```python
from build123d import *

# Parameters (mm, degrees)
SM_BASE_FLANGE_1_DEPTH = 30
SKETCH_6_R             = 1.7
CUT_EXTRUDE_1_DEPTH    = 10
SKETCH_7_R             = 1.7
CUT_EXTRUDE_2_DEPTH    = 10


# Sheet-metal steps are written as plain solids
with BuildPart() as part:
    # Sketch 1 → 基体-法兰1 (new body)
    with BuildSketch(Plane.XY):
        with BuildLine():
            Line((20, 0), (0.5, 0))
            ThreePointArc((0.5, 0), (0.146446609, 0.146446609), (0, 0.5))
            Line((0, 0.5), (0, 22))
            Line((0, 22), (-2, 22))
            Line((-2, 22), (-2, 0.5))
            ThreePointArc((-2, 0.5), (-1.267766953, -1.267766953), (0.5, -2))
            Line((0.5, -2), (20, -2))
            Line((20, -2), (20, 0))
        make_face()
    extrude(amount=SM_BASE_FLANGE_1_DEPTH)

    # 草图6 → 切除-拉伸1 (cut)
    with BuildSketch(Plane(origin=(0, 0, 0), x_dir=(0, 0, -1), z_dir=(1, 0, 0))):
        with Locations((-25, 18)):
            Circle(SKETCH_6_R)
        with Locations((-5, 18)):
            Circle(SKETCH_6_R)
    extrude(amount=-CUT_EXTRUDE_1_DEPTH, mode=Mode.SUBTRACT)

    # 草图7 → 切除-拉伸2 (cut)
    with BuildSketch(Plane(origin=(0, 0, 0), x_dir=(1, 0, 0), z_dir=(0, 1, 0))):
        with Locations(Location((16, -5, 0), (0, 0, 270))):
            Circle(SKETCH_7_R)
        with Locations(Location((16, -25, 0), (0, 0, 270))):
            Circle(SKETCH_7_R)
    extrude(amount=-CUT_EXTRUDE_2_DEPTH, mode=Mode.SUBTRACT)


solid = part.part
```
Work out the finished part from the listing and answer in its coordinate system (mm). A direction names the side the tool comes from. Round coordinates to 2 decimals unless told otherwise and drop trailing zeros. Loops run counter-clockwise (first coordinate to the right, second up) from the corner with the lowest first, then second, coordinate; pieces in that order, holes last.
(1) Find the intervals of material crossed by L1, parallel to X at y = 5.25, z = 15; L2, parallel to X at y = -0.7, z = 25, in increasing order.
Computed values:
L1: x = -2 to 0
L2: x = -1.69 to 14.3, 17.7 to 20
(2) The part is cut by section D-D, the plane z = 18.5. Give the vertices of the cut face in (x, y).
Computed values:
outline: (-2, 0.5) arc R2.5 ccw to (0.5, -2) - (20, -2) - (20, 0) - (0.5, 0) arc R0.5 cw to (0, 0.5) - (0, 22) - (-2, 22) - close
(3) For faces 1 (the flat face through (0, 11, 15)), 2 (the flat face through (-1, 22, 15)), determine the directions among +Z, -Z, +X, -X, +Y, -Y from which every point of the face is accessible in a straight line to the end or side of a thin tool.
Computed values:
face 1: +Z, -Z, +X, +Y
face 2: +Z, -Z, +X, -X, +Y
(4) The part is cut by section A-A, the plane y = 18. Give the vertices of the cut face in (x, z), and give its area (3 significant figures).
Computed values:
outline: (-2, 0) - (0, 0) - (0, 3.3) - (-2, 3.3) - close; (-2, 6.7) - (0, 6.7) - (0, 23.3) - (-2, 23.3) - close; (-2, 26.7) - (0, 26.7) - (0, 30) - (-2, 30) - close
area: 46.4 mm2
(5) The mould has two halves that part along Z. Classify faces 3 (the cylindrical face through (14.5, -1, 5.8)), 4 (the flat face through (10, 0, 15)), 5 (the cylindrical face through (-0.986, 19.686, 5.221)), 6 (the flat face through (-1, 7, 30)): pulls with the +Z half, pulls with the -Z half, needs draft (parallel to the pull), parting line crosses it, or undercut.
Computed values:
face 3: undercut
face 4: needs draft
face 5: undercut
face 6: pulls with the +Z half
(6) Each of these flat-tipped pins is pushed along its axis until it touches: P1, Ø6, axis at x = 10, z = 17, coming from the +Y side; P2, Ø4.5, axis at y = 18, z = 25, coming from the -X side; P3, Ø2, axis at y = 18, z = 5, coming from the +X side; P4, Ø8, axis at y = 13.5, z = 16.5, coming from the +X side. Where does it stop, or does it pass through?
Computed values:
P1: stops at y = 0
P2: stops at x = -2
P3: passes through
P4: stops at x = 0
(7) The part is cut by section C-C, the plane z = 5. Give the vertices of the cut face in (x, y), and give its area (3 significant figures).
Computed values:
outline: (-2, 0.5) arc R2.5 ccw to (0.5, -2) - (14.3, -2) - (14.3, 0) - (0.5, 0) arc R0.5 cw to (0, 0.5) - (0, 16.3) - (-2, 16.3) - close; (-2, 19.7) - (0, 19.7) - (0, 22) - (-2, 22) - close; (17.7, -2) - (20, -2) - (20, 0) - (17.7, 0) - close
area: 73.1 mm2
